from build123d import *

# Parameters (mm, degrees)
BOSS_EXTRUDE1_START = 1
SKETCH1_R           = 3.9
SKETCH1_R_2         = 1.4
BOSS_EXTRUDE1_DEPTH = 6
SKETCH2_R           = 5.3
SKETCH2_R_2         = 1.4
BOSS_EXTRUDE2_DEPTH = 3.4
CHAMFER1_SIZE       = 0.5
SKETCH3_R           = 2.2
CUT_EXTRUDE1_DEPTH  = 3.2
CHAMFER2_SIZE       = 1


with BuildPart() as part:
    # Sketch1 → Boss-Extrude1 (new body)
    with BuildSketch(Plane.XY.offset(BOSS_EXTRUDE1_START)):
        with Locations(Location((10.044784941, -1.265818107, 0), (0, 0, 180))):
            Circle(SKETCH1_R)
        with Locations(Location((10.044784941, -1.265818107, 0), (0, 0, 180))):
            Circle(SKETCH1_R_2, mode=Mode.SUBTRACT)
    extrude(amount=BOSS_EXTRUDE1_DEPTH)

    # Sketch2 → Boss-Extrude2 (add)
    with BuildSketch(Plane.XY.offset(7)):
        with Locations((10.044784941, -1.265818107)):
            Circle(SKETCH2_R)
        with Locations((10.044784941, -1.265818107)):
            Circle(SKETCH2_R_2, mode=Mode.SUBTRACT)
    extrude(amount=BOSS_EXTRUDE2_DEPTH)

    # Chamfer1
    chamfer1_edges = [part.edges().sort_by_distance(p)[0] for p in [
        (4.744784941, -1.265818107, 7),
    ]]
    chamfer(chamfer1_edges, length=CHAMFER1_SIZE)

    # Sketch3 → Cut-Extrude1 (cut)
    with BuildSketch(Plane.XY.offset(10.4)):
        with Locations((10.044784941, -1.265818107)):
            Circle(SKETCH3_R)
    extrude(amount=-CUT_EXTRUDE1_DEPTH, mode=Mode.SUBTRACT)

    # Chamfer2
    chamfer2_edges = [part.edges().sort_by_distance(p)[0] for p in [
        (13.944784941, -1.265818107, 1),
    ]]
    chamfer(chamfer2_edges, length=CHAMFER2_SIZE)


solid = part.part
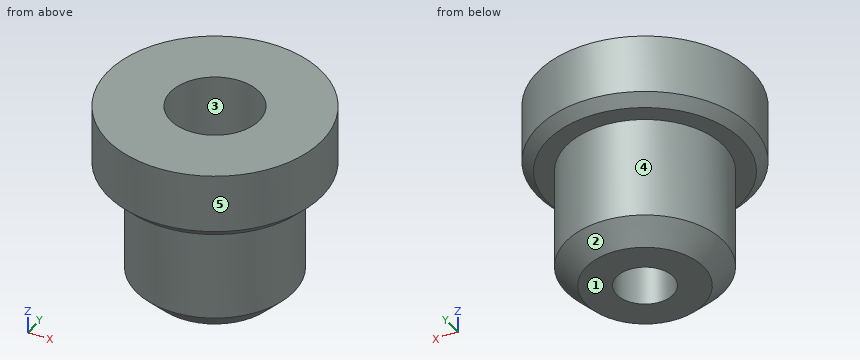
Geometry: final body of the model. Coordinates: model frame, mm. Face numbers are marked on the shaded views. A direction names the side the tool comes from. Coordinates: 2 decimals unless noted, no trailing zeros. Write each loop counter-clockwise with the first axis right and the second up, starting at its lowest first coordinate (ties: lowest second). Pieces come first, ordered by that corner, then holes. Notation, with made-up numbers: (77, 83) - (99, 83) arc R17 cw to (99, 100) - close; hole circle Ø10 at (-18.75, -33.75). An arc over 180 degrees is marked (long way). Return JSON: item names as keys, results as strings.
Item 1: Section query B-B (z = 9.25). Output: boundary loops of the cut face in (x, y).
Completed:
{"outline": "circle Ø10.6 at (10.04, -1.27); hole circle Ø4.4 at (10.04, -1.27)"}
Item 2: Pull-direction query (Y, two-part tool) for the marked faces 1, 2 and 3; classes: +Y half, -Y half, draft (parallel to the pull), parting line (faces both ways), or undercut.
Completed:
{"face 1": "draft", "face 2": "parting line", "face 3": "undercut"}
Item 3: Section query A-A (z = 6). Output: boundary loops of the cut face in (x, y).
Completed:
{"outline": "circle Ø7.8 at (10.04, -1.27); hole circle Ø2.8 at (10.04, -1.27)"}
Item 4: Reachability of the marked faces 4 and 5 from +Z, -Z, +X, -X, +Y, -Y: full face, straight path, thin tool, end or side. Return the list, or none.
Completed:
{"face 4": "-Z", "face 5": "+Z, -Z"}
Item 5: Line query: L1, parallel to Y at x = 9.75, z = 9.75; L2, parallel to Z at x = 13, y = 2.5; L3, parallel to X at y = -0.5, z = 7.25. Output: solid intervals per line, ascending.
Completed:
{"L1": "y = -6.56 to -3.45, 0.91 to 4.03", "L2": "z = 7 to 10.4", "L3": "x = 5.05 to 7.98, 12.11 to 15.04"}
Item 6: Pin query (flat end, axial travel): pin 1 Ø3.5 at (x, y) = (9.5, -1) entering from +Z; pin 2 Ø4 at (x, y) = (10.04, -1.27) entering from +Z; pin 3 Ø1.5 at (y, z) = (-2, 2.5) entering from -X; pin 4 Ø2 at (x, y) = (10.04, -1.27) entering from -Z. Return the tip coordinate at first contact, or that it passes through.
Completed:
{"pin 1": "stops at z = 10.4", "pin 2": "stops at z = 7.2", "pin 3": "stops at x = 6.14", "pin 4": "passes through"}
